Here's the drawing with two shaded views (mm, measured from the low corner). I have some questions. A direction names the side the tool comes from. Coordinates: 2 decimals unless noted, no trailing zeros. Write each loop counter-clockwise with the first axis right and the second up, starting at its lowest first coordinate (ties: lowest second). Pieces come first, ordered by that corner, then holes.
Item 1: I want a section at D-D on x = 4. Please give me the cut outline in (y, z), then the cut area to 4 significant figures.
Item 2: I want a section at B-B on z = 24. Please give me the cut outline in (x, y), then the cut area to 3 significant figures.
Item 3: I want a section at C-C on y = 8. Please give me the cut outline in (x, z), then the cut area to 3 significant figures.
Item 4: I want a section at A-A on x = 46. Please give me the cut outline in (y, z).
Item 5: Thinking about a two-plate mould opening in X: for the marked faces 3, 4 and 5, which applies, +X half, -X half, draft (parallel to the pull), parting line (faces both ways), or undercut?
Item 6: For P1, Ø1.9, axis at x = 12, y = 3, coming from the +Z side; P2, Ø2.5, axis at y = 3.5, z = 27, coming from the -X side; P3, Ø10, axis at x = 34.5, z = 19, coming from the -Y side; P4, Ø4, axis at x = 34, y = 1.5, coming from the +Z side, each with a flat end and sliding along its axis, tell me the tip position at first contact or that it passes through.
Item 7: Which directions (+Z, -Z, +X, -X, +Y, -Y) give clear straight access to the entire face, cutting with the end or side of a thin tool? Please do the marked faces 1 and 2.
Item 8: If I drill on probe 1 along X at (y, z) = (3.5, 22.5); probe 2 along X at (y, z) = (5.75, 30); probe 3 along Y at (x, z) = (46, 3.9), over which ranges is the centre line in solid material (lowest first)?
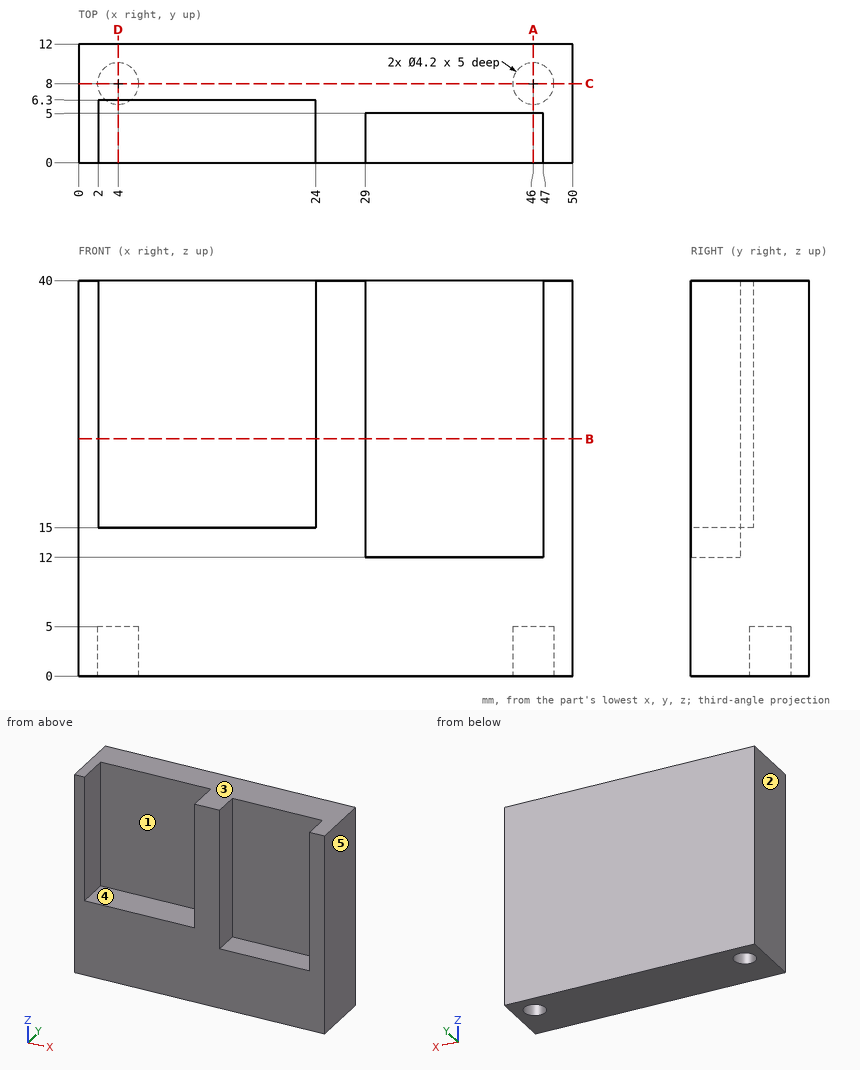
Response values:
1. outline: (0, 0) - (5.9, 0) - (5.9, 5) - (10.1, 5) - (10.1, 0) - (12, 0) - (12, 40) - (6.3, 40) - (6.3, 15) - (0, 15) - close
1. area: 301.5 mm2
2. outline: (0, 0) - (2, 0) - (2, 6.3) - (24, 6.3) - (24, 0) - (29, 0) - (29, 5) - (47, 5) - (47, 0) - (50, 0) - (50, 12) - (0, 12) - close
2. area: 371 mm2
3. outline: (0, 0) - (1.9, 0) - (1.9, 5) - (6.1, 5) - (6.1, 0) - (43.9, 0) - (43.9, 5) - (48.1, 5) - (48.1, 0) - (50, 0) - (50, 40) - (0, 40) - close
3. area: 1,960 mm2
4. outline: (0, 0) - (5.9, 0) - (5.9, 5) - (10.1, 5) - (10.1, 0) - (12, 0) - (12, 40) - (5, 40) - (5, 12) - (0, 12) - close
5. face 3: draft
5. face 4: undercut
5. face 5: +X half
6. P1: stops at z = 15
6. P2: stops at x = 0
6. P3: stops at y = 5
6. P4: stops at z = 12
7. face 1: +Z, -Y
7. face 2: +Z, -Z, -X, +Y, -Y
8. probe 1: x = 0 to 2, 24 to 29, 47 to 50
8. probe 2: x = 0 to 2, 24 to 50
8. probe 3: y = 0 to 5.9, 10.1 to 12
